The model under review builds one solid part; all positions refer to its coordinate system, in mm. A direction names the side the tool comes from. Round coordinates to 2 decimals unless told otherwise and drop trailing zeros. Order: outer loops, then holes, each group sorted by start corner. A loop starts at its lowest first (then second) coordinate and runs counter-clockwise, first axis right, second up.
```python
from build123d import *

# Parameters (mm, degrees)
SKETCH2_W           = 25.4
SKETCH2_H           = 25.4
BOSS_EXTRUDE1_DEPTH = 5.08
CUT_EXTRUDE1_DEPTH  = 5.08


with BuildPart() as part:
    # Sketch2 → Boss-Extrude1 (new body)
    with BuildSketch(Plane(origin=(0, 0, 0), x_dir=(1, 0, 0), z_dir=(0, 1, 0))):
        with Locations((12.7, 12.7)):
            Rectangle(SKETCH2_W, SKETCH2_H)
    extrude(amount=BOSS_EXTRUDE1_DEPTH)

    # Sketch3 → Cut-Extrude1 (cut)
    with BuildSketch(Plane(origin=(0, 5.08, 5.08), x_dir=(1, 0, 0), z_dir=(0, 1, 0))):
        with BuildLine():
            Line((6.35, 11.43), (8.957059761, 11.43))
            ThreePointArc((8.957059761, 11.43), (7.653529881, 13.6525), (6.35, 11.43))
        make_face()
        with BuildLine():
            Line((16.307858538, 11.43), (19.05, 11.43))
            ThreePointArc((19.05, 11.43), (17.678929269, 13.7795), (16.307858538, 11.43))
        make_face()
        with BuildLine():
            Line((6.35, 24.13), (8.872157331, 24.13))
            ThreePointArc((8.872157331, 24.13), (7.611078665, 26.289), (6.35, 24.13))
        make_face()
        with BuildLine():
            Line((16.375390855, 24.13), (19.05, 24.13))
            ThreePointArc((19.05, 24.13), (17.712695427, 26.416), (16.375390855, 24.13))
        make_face()
    extrude(amount=-CUT_EXTRUDE1_DEPTH, mode=Mode.SUBTRACT)


solid = part.part
```
(1) Consider section A-A (y = 4.05). Write out the cut boundary in (x, z).
Data:
outline: (0, -25.4) - (25.4, -25.4) - (25.4, 0) - (0, 0) - close; hole (6.35, -19.05) arc R1.45 ccw (long way) to (8.87, -19.05) - close; hole (6.35, -6.35) arc R1.49 ccw (long way) to (8.96, -6.35) - close; hole (16.31, -6.35) arc R1.57 ccw (long way) to (19.05, -6.35) - close; hole (16.38, -19.05) arc R1.53 ccw (long way) to (19.05, -19.05) - close
(2) For faces 1 (the flat face through (13, 0, -13)), 2 (the flat face through (18, 3, -19.05)), list the 3-axis set-ups (+Z, -Z, +X, -X, +Y, -Y) from which the entire face can be reached by the end or side of a thin tool; tool diameter is ignored.
Data:
face 1: +Z, -Z, +X, -X, -Y
face 2: +Y, -Y
(3) Consider section B-B (x = 18). Write out the cut boundary in (y, z), and give its area (3 significant figures).
Data:
outline: (0, -25.4) - (5.08, -25.4) - (5.08, -21.31) - (0, -21.31) - close; (0, -19.05) - (5.08, -19.05) - (5.08, -8.67) - (0, -8.67) - close; (0, -6.35) - (5.08, -6.35) - (5.08, 0) - (0, 0) - close
area: 106 mm2
(4) Draft analysis for pull direction Z (two halves, no side actions). For faces 3 (the cylindrical face through (17.757, 2.576, -21.335)), 4 (the flat face through (13, 5.08, -13)), 5 (the flat face through (13, 3, -25.4)), 6 (the flat face through (13, 3, 0)), state which applies: pulls with the +Z half, pulls with the -Z half, needs draft (parallel to the pull), parting line crosses it, or undercut.
Data:
face 3: undercut
face 4: needs draft
face 5: pulls with the -Z half
face 6: pulls with the +Z half
(5) Insertion check: pin 1 (5 mm diameter, centred on x = 7.65, z = -7.08, fed in from -Y). The pin has a flat end and moves straight along its axis. Give the tip position at first contact, or say it passes through.
Data:
pin 1: stops at y = 0
